```python
from build123d import *

# Parameters (mm, degrees)
SKETCH1_R           = 360
BOSS_EXTRUDE1_DEPTH = 60
SKETCH2_R           = 358
SKETCH2_R_2         = 150
CUT_EXTRUDE1_DEPTH  = 50
SKETCH3_W           = 19.673543
SKETCH3_H           = 15
CUT_EXTRUDE2_DEPTH  = 160
MOVE_FACE1_BY       = 30
FILLET1_R           = 6


with BuildPart() as part:
    # Sketch1 → Boss-Extrude1 (new body)
    with BuildSketch(Plane(origin=(0, 0, 0), x_dir=(1, 0, 0), z_dir=(0, 1, 0))):
        with Locations(Location((0, 0, 0), (0, 0, 270))):
            Circle(SKETCH1_R)
    extrude(amount=BOSS_EXTRUDE1_DEPTH)

    # Sketch2 → Cut-Extrude1 (cut)
    with BuildSketch(Plane(origin=(0, 60, 0), x_dir=(1, 0, 0), z_dir=(0, 1, 0))):
        with Locations(Location((0, 0, 0), (0, 0, 270))):
            Circle(SKETCH2_R)
        with Locations(Location((0, 0, 0), (0, 0, 270))):
            Circle(SKETCH2_R_2, mode=Mode.SUBTRACT)
    extrude(amount=-CUT_EXTRUDE1_DEPTH, mode=Mode.SUBTRACT)

    # Sketch3 → Cut-Extrude2 (cut)
    with BuildSketch(Plane.XY.offset(360)):
        with Locations((27.8367715, 7.5)):
            Rectangle(SKETCH3_W, SKETCH3_H)
    extrude(amount=-CUT_EXTRUDE2_DEPTH, mode=Mode.SUBTRACT)

    # Move Face1: a face moved inward by 30.0
    extrude(part.faces().sort_by_distance((0, 60, 0))[0], amount=MOVE_FACE1_BY, dir=(0, -1, 0), mode=Mode.SUBTRACT)

    # Fillet1
    fillet1_edges = [part.edges().sort_by_distance(p)[0] for p in [
        (18, 5, 200),
        (37.673543, 5, 200),
    ]]
    fillet(fillet1_edges, radius=FILLET1_R)


solid = part.part
```
Here's how the part is built. I have some questions about the finished solid (model axes, mm). Coordinates: 2 decimals unless noted, no trailing zeros. Write each loop counter-clockwise with the first axis right and the second up, starting at its lowest first coordinate (ties: lowest second). Pieces come first, ordered by that corner, then holes. Notation, with made-up numbers: M 49,81.5 L 70,81.5 A10 ccw 70,93.5 Z; hole C 89.25,33.25 d3. An arc over 180 degrees is marked long. Answer as CSV lines item,"result". Start each with the question number.
Q1. Will these pins go through, and if not, where does the flat tip stop? pin 1 Ø12 at (y, z) = (5, 311) entering from +X; pin 2 Ø7.5 at (y, z) = (7, 292.5) entering from -X; pin 3 Ø12 at (y, z) = (9, -73) entering from -X.
Q2. Suppose I cut it at D-D, the plane z = -194. List the corners of the cut face in (x, y) for me.
Q3. Suppose I cut it at A-A, the plane y = 51. List the corners of the cut face in (x, z) for me.
Q4. If we mould it in two halves opening along X, with no side actions, what happens to faces 1 (the cylindrical face through (-91.273, 20.14, -119.035)), 2 (the cylindrical face through (-349.487, 35.35, -77.607)), 3 (the cylindrical face through (-137.88, 29.58, 332.55)), 4 (the flat face through (5, 0, -5))? For each: pulls with the +X half, pulls with the -X half, needs draft (parallel to the pull), parting line crosses it, or undercut.
Q5. Suppose I cut it at C-C, the plane x = 0. List the corners of the cut face in (y, z) for me, then the cut area to 3 significant figures.
Q6. Suppose I cut it at B-B, the plane z = -39. List the corners of the cut face in (x, y) for me, then the cut area to 3 significant figures.
Q7. I need wall thicknesses on probe 1 along Z at (x, y) = (0, 49.5); probe 2 along X at (y, z) = (27.5, 0). Which ranges of each line are inside material? Lowest first, please. Write a range as [from, to].
Entries:
1,pin 1,"stops at x = 191.25"
1,pin 2,"stops at x = -215"
1,pin 3,"stops at x = -353.71"
2,outline,"M -303.26,0 L 303.26,0 L 303.26,60 L 300.88,60 L 300.88,10 L -300.88,10 L -300.88,60 L -303.26,60 Z"
3,outline,"C 0,0 d720; hole C 0,0 d716"
4,face 1,"undercut"
4,face 2,"undercut"
4,face 3,"parting line crosses it"
4,face 4,"needs draft"
5,outline,"M 0,-360 L 60,-360 L 60,-358 L 10,-358 L 10,-150 L 30,-150 L 30,150 L 10,150 L 10,358 L 60,358 L 60,360 L 0,360 Z"
5,area,"13,400 mm²"
6,outline,"M -357.88,0 L 357.88,0 L 357.88,60 L 355.87,60 L 355.87,10 L 144.84,10 L 144.84,30 L -144.84,30 L -144.84,10 L -355.87,10 L -355.87,60 L -357.88,60 Z"
6,area,"13,200 mm²"
7,probe 1,"z = [-360, -358], [358, 360]"
7,probe 2,"x = [-360, -358], [-150, 150], [358, 360]"
